Source: three-view drawing plus pictorial views. Frame: mm from the lowest corner of the part. Coordinates: 2 decimals unless noted, no trailing zeros. Write each loop counter-clockwise with the first axis right and the second up, starting at its lowest first coordinate (ties: lowest second). Pieces come first, ordered by that corner, then holes. Notation, with made-up numbers: (0.25, -7) - (59.25, -7) arc R31 cw to (59.25, 28) - close; hole circle Ø10 at (85.25, -28.75). An arc over 180 degrees is marked (long way). Put each result on its own line as item: value.
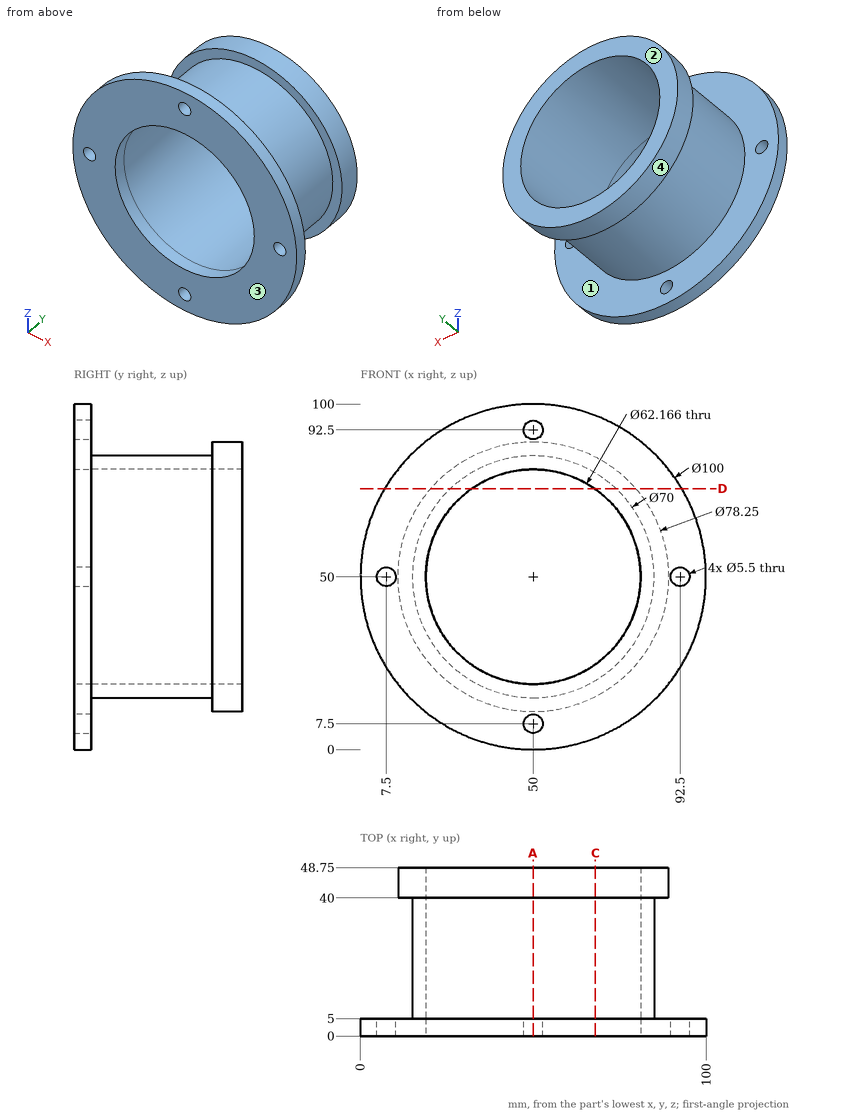
1. Section query A-A (x = 50). Count the separate pieces of the cut face and the enclosed holes in it, then the cut area to 3 significant figures.
Answer below:
separate pieces: 4
enclosed holes: 0
area: 549 mm²
2. Section query D-D (z = 75.5). Return loops of the section in (x, y).
Answer below:
outline: (6.99, 0) - (32.23, 0) - (32.23, 48.75) - (20.33, 48.75) - (20.33, 40) - (26.03, 40) - (26.03, 5) - (6.99, 5) - close; (67.77, 0) - (93.01, 0) - (93.01, 5) - (73.97, 5) - (73.97, 40) - (79.67, 40) - (79.67, 48.75) - (67.77, 48.75) - close
3. Pin query (flat end, axial travel): pin 1 Ø2 at (y, z) = (27, 61) entering from -X; pin 2 Ø3 at (x, y) = (57, 28.5) entering from -Z (1 decimal); pin 3 Ø8 at (y, z) = (28.5, 81.5) entering from +X. Return the tip coordinate at first contact, or that it passes through.
Answer below:
pin 1: stops at x = 16.46
pin 2: stops at z = 15.4
pin 3: stops at x = 71.65
4. Ray query, probe 1 along X at (y, z) = (1.2, 50); probe 2 along Y at (x, z) = (87.5, 40); probe 3 along Y at (x, z) = (88.5, 24.5). Return the intervals inside material, ascending. Write a range as from..to.
Answer below:
probe 1: x = 0..4.75, 10.25..18.92, 81.08..89.75, 95.25..100
probe 2: y = 0..5, 40..48.75
probe 3: y = 0..5
5. Section query C-C (x = 68). Return loops of the section in (y, z), then the cut area to 3 significant figures.
Answer below:
outline: (0, 3.35) - (5, 3.35) - (5, 19.98) - (40, 19.98) - (40, 15.26) - (48.75, 15.26) - (48.75, 24.66) - (0, 24.66) - close; (0, 75.34) - (48.75, 75.34) - (48.75, 84.74) - (40, 84.74) - (40, 80.02) - (5, 80.02) - (5, 96.65) - (0, 96.65) - close
area: 705 mm²
6. Mould query, pull axis Y, two halves, no side actions, for the marked faces 1, 2, 3 and 4. Classes: +Y half, -Y half, draft (parallel to the pull), parting line (faces both ways), or undercut.
Answer below:
face 1: undercut
face 2: +Y half
face 3: -Y half
face 4: draft
